Design review of the part shown in the three views and the two pictorial views. Dimensions are in mm from the part's minimum x, y and z. Coordinates: 2 decimals unless noted, no trailing zeros. Write each loop counter-clockwise with the first axis right and the second up, starting at its lowest first coordinate (ties: lowest second). Pieces come first, ordered by that corner, then holes.
Q1. For pin 1 Ø1.5 at (y, z) = (80, 5.5) entering from +X; pin 2 Ø1 at (x, y) = (350.5, 66.5) entering from -Z; pin 3 Ø6.5 at (x, z) = (604, 3.5) entering from -Y; pin 4 Ø4 at (y, z) = (8.5, 4.5) entering from -X, all flat-tipped, find the tip position at first contact; note any pin that passes through.
Q2. For L1, parallel to Y at x = 193, z = 2; L2, parallel to X at y = 84.5, z = 6.25; L3, parallel to Z at x = 96, y = 16, list the stretches that pass through material, from the lowest coordinate up.
Q3. Take a section at B-B, the plane x = 509.5. Write out the cut boundary in (y, z).
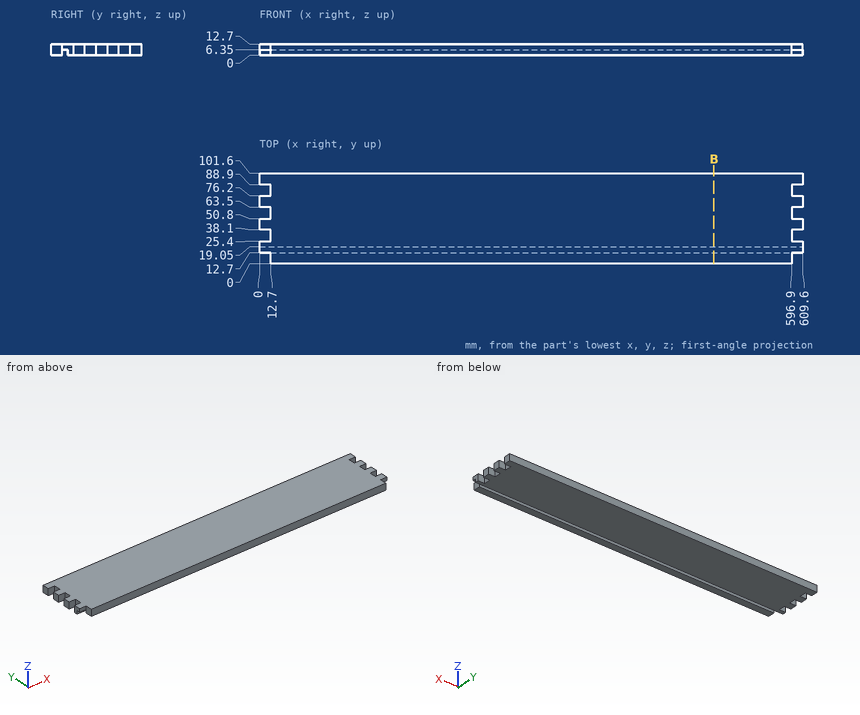
Responses:
1. pin 1: stops at x = 596.9
1. pin 2: stops at z = 0
1. pin 3: stops at y = 12.7
1. pin 4: stops at x = 12.7
2. L1: y = 0 to 12.7, 19.05 to 101.6
2. L2: x = 12.7 to 596.9
2. L3: z = 6.35 to 12.7
3. outline: (0, 0) - (12.7, 0) - (12.7, 6.35) - (19.05, 6.35) - (19.05, 0) - (101.6, 0) - (101.6, 12.7) - (0, 12.7) - close
